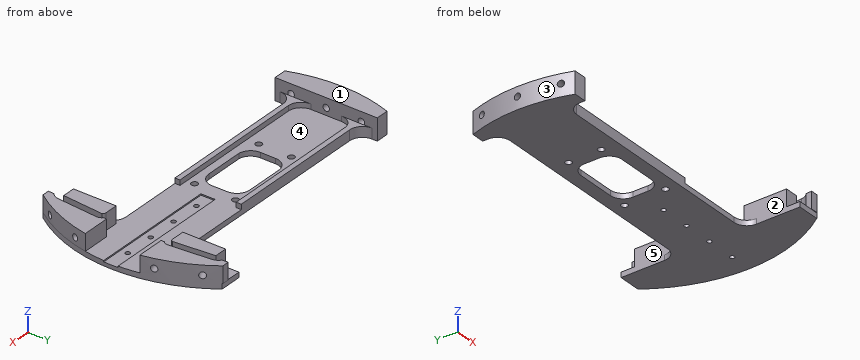
from build123d import *

# Parameters (mm, degrees)
SKETCH1_R           = 1.5875
BOSS_EXTRUDE1_DEPTH = 2.54
BOSS_EXTRUDE2_DEPTH = 8.255
SKETCH3_W           = 64.77
SKETCH3_H           = 7.1
CUT_EXTRUDE1_DEPTH  = 0.635
SKETCH9_R           = 1.5875
CUT_EXTRUDE4_DEPTH  = 3.54
SKETCH4_R           = 1.143
CUT_EXTRUDE2_DEPTH  = 11.43
BOSS_EXTRUDE5_DEPTH = 8.255
SKETCH28_R          = 1.5875
CUT_EXTRUDE12_DEPTH = 7.62
SKETCH29_R          = 1.5875
CUT_EXTRUDE13_DEPTH = 10.16
SKETCH30_R          = 1.5875
CUT_EXTRUDE14_DEPTH = 12.7
SKETCH31_R          = 1.5875
CUT_EXTRUDE15_DEPTH = 12.7
SKETCH32_R          = 1.5875
CUT_EXTRUDE16_DEPTH = 12.7
BOSS_EXTRUDE6_DEPTH = 2.54
CUT_EXTRUDE17_DEPTH = 3.5400001


with BuildPart() as part:
    # Sketch1 → Boss-Extrude1 (new body)
    with BuildSketch(Plane.XY):
        with BuildLine():
            Line((-71.572584947, 25.4), (-65.222584947, 25.4))
            Line((-65.222584947, 25.4), (-65.222584947, 22.86))
            ThreePointArc((-65.222584947, 22.86), (-63.362713008, 18.369871939), (-58.872584947, 16.51))
            Line((-58.872584947, 16.51), (44.196, 16.51))
            ThreePointArc((44.196, 16.51), (48.686128061, 18.369871939), (50.546, 22.86))
            Line((50.546, 22.86), (50.546, 44.45))
            Line((50.546, 44.45), (61.579155694, 44.45))
            ThreePointArc((61.579155694, 44.45), (75.946, 0), (61.579155694, -44.45))
            Line((61.579155694, -44.45), (50.546, -44.45))
            Line((50.546, -44.45), (50.546, -22.86))
            ThreePointArc((50.546, -22.86), (48.686128061, -18.369871939), (44.196, -16.51))
            Line((44.196, -16.51), (-58.872584947, -16.51))
            ThreePointArc((-58.872584947, -16.51), (-63.362713008, -18.369871939), (-65.222584947, -22.86))
            Line((-65.222584947, -22.86), (-65.222584947, -25.4))
            Line((-65.222584947, -25.4), (-71.572584947, -25.4))
            ThreePointArc((-71.572584947, -25.4), (-75.946, 0), (-71.572584947, 25.4))
        make_face()
        with Locations((-31.75, 8.128)):
            Circle(SKETCH1_R, mode=Mode.SUBTRACT)
        with Locations((-31.75, -8.128)):
            Circle(SKETCH1_R, mode=Mode.SUBTRACT)
    extrude(amount=BOSS_EXTRUDE1_DEPTH)

    # Sketch2 → Boss-Extrude2 (add)
    with BuildSketch(Plane.XY.offset(2.54)):
        with BuildLine():
            Line((61.865268471, 17.78), (60.095110466, 38.1))
            ThreePointArc((60.095110466, 38.1), (59.464196764, 40.158289632), (58.047089349, 41.778911391))
            Line((58.047089349, 41.778911391), (57.900800643, 44.704))
            Line((57.900800643, 44.704), (61.395010384, 44.704))
            ThreePointArc((61.395010384, 44.704), (69.822038137, 29.877715884), (74.728381149, 13.544887112))
            Line((74.728381149, 13.544887112), (60.759450402, 13.544887112))
            Line((60.759450402, 13.544887112), (60.759450402, 15.094127876))
            ThreePointArc((60.759450402, 15.094127876), (61.639191639, 16.302501703), (61.865268471, 17.78))
        make_face()
        with BuildLine():
            Line((58.651639318, 17.500047669), (56.881481313, 37.820047669))
            Line((56.881481313, 37.820047669), (50.546, 37.820047669))
            Line((50.546, 37.820047669), (50.546, 16.566735288))
            Line((50.546, 16.566735288), (57.366094516, 16.566735288))
            ThreePointArc((57.366094516, 16.566735288), (58.160401987, 16.824667019), (58.651639318, 17.500047669))
        make_face()
        with BuildLine():
            Line((60.759450402, -13.544887112), (74.728381149, -13.544887112))
            ThreePointArc((74.728381149, -13.544887112), (69.822038137, -29.877715884), (61.395010384, -44.704))
            Line((61.395010384, -44.704), (57.900800643, -44.704))
            Line((57.900800643, -44.704), (58.047089349, -41.778911391))
            ThreePointArc((58.047089349, -41.778911391), (59.464196764, -40.158289632), (60.095110466, -38.1))
            Line((60.095110466, -38.1), (61.865268471, -17.78))
            ThreePointArc((61.865268471, -17.78), (61.639191639, -16.302501703), (60.759450402, -15.094127876))
            Line((60.759450402, -15.094127876), (60.759450402, -13.544887112))
        make_face()
        with BuildLine():
            Line((50.546, -16.566735288), (57.366094516, -16.566735288))
            ThreePointArc((57.366094516, -16.566735288), (58.160401987, -16.824667019), (58.651639318, -17.500047669))
            Line((58.651639318, -17.500047669), (56.881481313, -37.820047669))
            Line((56.881481313, -37.820047669), (50.546, -37.820047669))
            Line((50.546, -37.820047669), (50.546, -16.566735288))
        make_face()
    extrude(amount=BOSS_EXTRUDE2_DEPTH)

    # Sketch3 → Cut-Extrude1 (cut)
    with BuildSketch(Plane.XY.offset(2.54)):
        with Locations((44.577, 0)):
            Rectangle(SKETCH3_W, SKETCH3_H)
    extrude(amount=-CUT_EXTRUDE1_DEPTH, mode=Mode.SUBTRACT)

    # Sketch9 → Cut-Extrude4 (cut, through all)
    with BuildSketch(Plane.XY.offset(2.54)):
        with Locations((7.62, -10.16)):
            Circle(SKETCH9_R)
        with Locations((7.62, 10.16)):
            Circle(SKETCH9_R)
    extrude(amount=-CUT_EXTRUDE4_DEPTH, mode=Mode.SUBTRACT)

    # Sketch4 → Cut-Extrude2 (cut)
    with BuildSketch(Plane.XY.offset(1.905)):
        with Locations((19.812, 0)):
            Circle(SKETCH4_R)
        with Locations((34.798, 0)):
            Circle(SKETCH4_R)
        with Locations((49.784, 0)):
            Circle(SKETCH4_R)
        with Locations((64.77, 0)):
            Circle(SKETCH4_R)
    extrude(amount=-CUT_EXTRUDE2_DEPTH, mode=Mode.SUBTRACT)

    # Sketch19 → Boss-Extrude5 (add)
    with BuildSketch(Plane.XY.offset(2.54)):
        with BuildLine():
            Line((-71.572584947, -25.4), (-65.222584947, -25.4))
            Line((-65.222584947, -25.4), (-65.222584947, 25.4))
            Line((-65.222584947, 25.4), (-71.572584947, 25.4))
            ThreePointArc((-71.572584947, 25.4), (-75.946, 0), (-71.572584947, -25.4))
        make_face()
    extrude(amount=BOSS_EXTRUDE5_DEPTH)

    # Sketch28 → Cut-Extrude12 (cut)
    with BuildSketch(Plane(origin=(65.771165316, 37.973, 0), x_dir=(0, 0, -1), z_dir=(0.866025404, 0.5, 0))):
        with Locations((-6.053310192, 0)):
            Circle(SKETCH28_R)
    cut_extrude12 = extrude(amount=-CUT_EXTRUDE12_DEPTH, mode=Mode.SUBTRACT)

    # Sketch29 → Cut-Extrude13 (cut)
    with BuildSketch(Plane(origin=(73.358202803, 19.656271199, 0), x_dir=(0, 0, -1), z_dir=(0.965925826, 0.258819045, 0))):
        with Locations((-6.096, 0)):
            Circle(SKETCH29_R)
    cut_extrude13 = extrude(amount=-CUT_EXTRUDE13_DEPTH, mode=Mode.SUBTRACT)

    # Mirror3: Cut-Extrude12, Cut-Extrude13 across plane
    add(cut_extrude12.mirror(Plane.ZX), mode=Mode.SUBTRACT)
    add(cut_extrude13.mirror(Plane.ZX), mode=Mode.SUBTRACT)

    # Sketch30 → Cut-Extrude14 (cut)
    with BuildSketch(Plane(origin=(-73.358202803, 19.656271199, 0), x_dir=(0, 0, 1), z_dir=(-0.965925826, 0.258819045, 0))):
        with Locations((6.096, 0)):
            Circle(SKETCH30_R)
    extrude(amount=-CUT_EXTRUDE14_DEPTH, mode=Mode.SUBTRACT)

    # Sketch31 → Cut-Extrude15 (cut)
    with BuildSketch(Plane.ZY.offset(75.946)):
        with Locations((6.096, 0)):
            Circle(SKETCH31_R)
    extrude(amount=-CUT_EXTRUDE15_DEPTH, mode=Mode.SUBTRACT)

    # Sketch32 → Cut-Extrude16 (cut)
    with BuildSketch(Plane(origin=(-73.358202803, -19.656271199, 0), x_dir=(0, 0, 1), z_dir=(-0.965925826, -0.258819045, 0))):
        with Locations((6.096, 0)):
            Circle(SKETCH32_R)
    extrude(amount=-CUT_EXTRUDE16_DEPTH, mode=Mode.SUBTRACT)

    # Sketch33 → Boss-Extrude6 (add)
    with BuildSketch(Plane.XY.offset(2.54)):
        with BuildLine():
            Line((12.137284041, 16.51), (-58.872584947, 16.51))
            ThreePointArc((-58.872584947, 16.51), (-63.362713008, 18.369871939), (-65.222584947, 22.86))
            Line((-65.222584947, 22.86), (-65.222584947, 7.62))
            ThreePointArc((-65.222584947, 7.62), (-63.362713008, 12.110128061), (-58.872584947, 13.97))
            Line((-58.872584947, 13.97), (12.137284041, 13.97))
            Line((12.137284041, 13.97), (12.137284041, 16.51))
        make_face()
        with BuildLine():
            Line((12.137284041, -13.97), (12.137284041, -16.51))
            Line((12.137284041, -16.51), (-58.872584947, -16.51))
            ThreePointArc((-58.872584947, -16.51), (-63.362713008, -18.369871939), (-65.222584947, -22.86))
            Line((-65.222584947, -22.86), (-65.222584947, -7.62))
            ThreePointArc((-65.222584947, -7.62), (-63.362713008, -12.110128061), (-58.872584947, -13.97))
            Line((-58.872584947, -13.97), (12.137284041, -13.97))
        make_face()
    extrude(amount=BOSS_EXTRUDE6_DEPTH)

    # Sketch34 → Cut-Extrude17 (cut, through all)
    with BuildSketch(Plane.XY.offset(2.54)):
        with BuildLine():
            Line((-20.772584947, 10.16), (-1.722584947, 10.16))
            ThreePointArc((-1.722584947, 10.16), (2.767543114, 8.300128061), (4.627415053, 3.81))
            Line((4.627415053, 3.81), (4.627415053, -3.81))
            ThreePointArc((4.627415053, -3.81), (2.767543114, -8.300128061), (-1.722584947, -10.16))
            Line((-1.722584947, -10.16), (-21.339131073, -10.16))
            ThreePointArc((-21.339131073, -10.16), (-25.458738375, -8.120468891), (-27.122584947, -3.83532408))
            Line((-27.122584947, -3.83532408), (-27.122584947, 3.81))
            ThreePointArc((-27.122584947, 3.81), (-25.262713008, 8.300128061), (-20.772584947, 10.16))
        make_face()
    extrude(amount=-CUT_EXTRUDE17_DEPTH, mode=Mode.SUBTRACT)


solid = part.part
For this review, take the finished solid that the model builds, in its own axes (mm). Face numbers are marked on the shaded views. A direction names the side the tool comes from. Give positions to 0.01 mm unless a question says otherwise; leave off trailing zeros. Loops run counter-clockwise (first coordinate to the right, second up) from the corner with the lowest first, then second, coordinate; pieces in that order, holes last. Notation, with made-up numbers: M -32.75,84 L -24.75,84 A15 ccw -24.75,105 Z; hole C 25.5,43 d9. An arc over 180 degrees is marked long. Answer as a JSON object with one key per item and string values. Group by question number.
Q1. Tool access review of the marked faces 1 and 2: name each direction out of +Z, -Z, +X, -X, +Y, -Y from which nothing blocks a thin tool from reaching the whole face with its end or side.
Q2. For probe 1 along Y at (x, z) = (-31.75, 1.8); probe 2 along Y at (x, z) = (-2, 2.5); probe 3 along Y at (x, z) = (56, 10.25), list the stretches that pass through material, from the lowest coordinate up. Write a range as [from, to].
Q3. Add section C-C on y = -31. Give the boundary of the cut face in (x, z) (3 decimals).
Q4. Insertion check: P1, Ø0.7, axis at x = 46, z = 2, coming from the -Y side; P2, Ø3.5, axis at x = 55, z = 7, coming from the +Y side; P3, Ø3, axis at y = 4, z = 2, coming from the -X side. Each pin has a flat end and moves straight along its axis. Give the tip position at first contact, or say it passes through.
Q5. Mouldability with a two-part tool opening along Y and no side actions: class the marked faces 3, 4 and 5 as +Y half, -Y half, draft (parallel to the pull), parting line (faces both ways), or undercut.
Q6. Add section D-D on x = 53. Give the boundary of the cut face in (y, z) (3 decimals), and give its area (3 significant figures).
Q7. Add section B-B on x = -18. Give the boundary of the cut face in (y, z).
Q8. Add section A-A on x = 7.62. Give the boundary of the cut face in (y, z), and give its area (3 significant figures).
Checked values:
{
 "1": {"face 1": "+Z, +X, -X, +Y, -Y", "face 2": "+Z, -Y"},
 "2": {"probe 1": "[-16.51, -9.72], [-6.54, 6.54], [9.72, 16.51]", "probe 2": "[-16.51, -10.16], [10.16, 16.51]", "probe 3": "[-37.82, -16.57], [16.57, 37.82]"},
 "3": {"outline": "M 50.546,0 L 69.331,0 L 69.331,10.795 L 60.714,10.795 L 60.714,2.54 L 57.476,2.54 L 57.476,10.795 L 50.546,10.795 Z"},
 "4": {"P1": "y = -16.89", "P2": "y = 37.82", "P3": "x = -75.9"},
 "5": {"face 3": "parting line", "face 4": "undercut", "face 5": "draft"},
 "6": {"outline": "M -44.45,0 L 44.45,0 L 44.45,2.54 L 37.82,2.54 L 37.82,10.795 L 16.567,10.795 L 16.567,2.54 L 3.55,2.54 L 3.55,1.905 L -3.55,1.905 L -3.55,2.54 L -16.567,2.54 L -16.567,10.795 L -37.82,10.795 L -37.82,2.54 L -44.45,2.54 Z", "area": "572 mm²"},
 "7": {"outline": "M -16.51,0 L -10.16,0 L -10.16,2.54 L -13.97,2.54 L -13.97,5.08 L -16.51,5.08 Z; M 10.16,0 L 16.51,0 L 16.51,5.08 L 13.97,5.08 L 13.97,2.54 L 10.16,2.54 Z"},
 "8": {"outline": "M -16.51,0 L -11.75,0 L -11.75,2.54 L -13.97,2.54 L -13.97,5.08 L -16.51,5.08 Z; M -8.57,0 L 8.57,0 L 8.57,2.54 L -8.57,2.54 Z; M 11.75,0 L 16.51,0 L 16.51,5.08 L 13.97,5.08 L 13.97,2.54 L 11.75,2.54 Z", "area": "80.6 mm²"}
}
